from build123d import *

# Parameters (mm, degrees)
SKETCH1_R           = 10
BOSS_EXTRUDE1_DEPTH = 0.79375
CUT_EXTRUDE3_DEPTH  = 27.174988807
FILLET1_R           = 5


with BuildPart() as part:
    # Sketch1 → Boss-Extrude1 (new body)
    # profile 1 of 2: a face of its own
    with BuildSketch(Plane.XY):
        with BuildLine():
            Line((12, -14.08012784), (12, 14.08012784))
            ThreePointArc((12, 14.08012784), (-18.5, 0), (12, -14.08012784))
        make_face()
        Circle(SKETCH1_R, mode=Mode.SUBTRACT)
    # profile 2 of 2: a face of its own
    with BuildSketch(Plane.XY):
        with BuildLine():
            ThreePointArc((18.5, 0), (16.796577032, 7.75403121), (12, 14.08012784))
            Line((12, 14.08012784), (12, -14.08012784))
            ThreePointArc((12, -14.08012784), (16.796577032, -7.75403121), (18.5, 0))
        make_face()
    extrude(amount=BOSS_EXTRUDE1_DEPTH)

    # Sketch1_3 → Cut-Extrude3 (cut, through all)
    with BuildSketch(Plane.XY):
        with BuildLine():
            ThreePointArc((18.5, 0), (16.796577032, 7.75403121), (12, 14.08012784))
            Line((12, 14.08012784), (12, -14.08012784))
            ThreePointArc((12, -14.08012784), (16.796577032, -7.75403121), (18.5, 0))
        make_face()
    extrude(amount=CUT_EXTRUDE3_DEPTH, mode=Mode.SUBTRACT)

    # Fillet1
    fillet1_edges = [part.edges().sort_by_distance(p)[0] for p in [
        (12, 14.08012784, 0.396875),
        (12, -14.08012784, 0.396875),
    ]]
    fillet(fillet1_edges, radius=FILLET1_R)


solid = part.part
Part model, mm, in its own coordinate system. Round coordinates to 2 decimals unless told otherwise and drop trailing zeros. Write each loop counter-clockwise with the first axis right and the second up, starting at its lowest first coordinate (ties: lowest second). Pieces come first, ordered by that corner, then holes. Notation, with made-up numbers: M 24.25,57 L 57.25,57 A16 ccw 57.25,73 Z; hole C 17.25,-6 d3. An arc over 180 degrees is marked long. Return JSON: item names as keys, results as strings. Group by question number.
(1) Saw through at B-B on y = 0. Write the cut outline in (x, z), then the cut area to 3 significant figures.
(2) Drill centre lines: probe 1 along Y at (x, z) = (0, 0.65); probe 2 along X at (y, z) = (-7, 0.75); probe 3 along Y at (x, z) = (-5, 0.15). Where is each one in solid material? Low to high.
(3) Two-plate mould, pull along X, no slides. Class faces 1 (the face through (11.34, -14.03, 0.4)), 2 (the face through (-10.2, 0.3, 0)), 3 (the face through (-2.17, -9.76, 0.39)): +X half, -X half, draft (parallel to the pull), parting line (faces both ways), or undercut.
(4) Saw through at A-A on x = 0. Write the cut outline in (y, z).
(5) Saw through at D-D on x = -11. Write the cut outline in (y, z), then the cut area to 3 significant figures.
(6) Saw through at C-C on z = 0.4. Write the cut outline in (x, y).
Returned:
{
 "1": {"outline": "M -18.5,0 L -10,0 L -10,0.79 L -18.5,0.79 Z; M 10,0 L 12,0 L 12,0.79 L 10,0.79 Z", "area": "8.33 mm²"},
 "2": {"probe 1": "-18.5 to -10, 10 to 18.5", "probe 2": "-17.12 to -7.14, 7.14 to 12", "probe 3": "-17.81 to -8.66, 8.66 to 17.81"},
 "3": {"face 1": "+X half", "face 2": "draft", "face 3": "undercut"},
 "4": {"outline": "M -18.5,0 L -10,0 L -10,0.79 L -18.5,0.79 Z; M 10,0 L 18.5,0 L 18.5,0.79 L 10,0.79 Z"},
 "5": {"outline": "M -14.87,0 L 14.87,0 L 14.87,0.79 L -14.87,0.79 Z", "area": "23.6 mm²"},
 "6": {"outline": "M 9.59,-15.82 A5 ccw 12,-11.54 L 12,11.54 A5 ccw 9.59,15.82 A18.5 ccw long Z; hole C 0,0 d20"}
}
